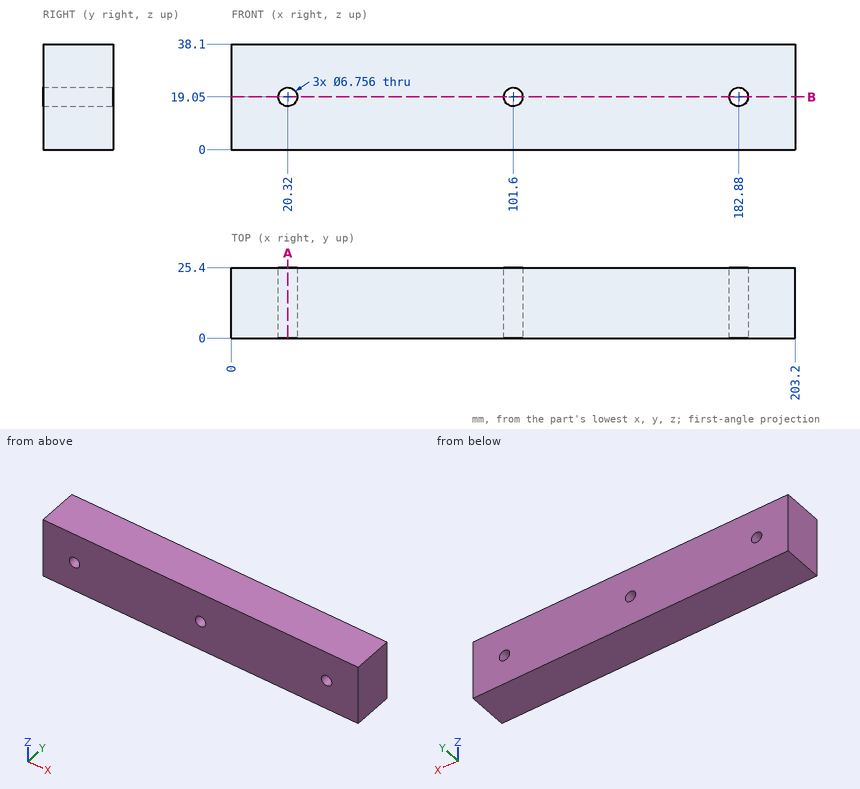
Job drawing, mm, ordinate dimensions from the low corner. One solid piece. Coordinates: 2 decimals unless noted, no trailing zeros. Order: outer loops, then holes, each group sorted by start corner. A loop starts at its lowest first (then second) coordinate and runs counter-clockwise, first axis right, second up. Notation, with made-up numbers: (46, 82) - (58, 82) arc R19 ccw to (58, 99) - close; hole circle Ø1 at (33, 53.25). An arc over 180 degrees is marked (long way). Return JSON: item names as keys, results as strings. Group by question number.
1) Probe line 1 (X direction, y = 13.25, z = 19.05); line 2 (Z direction, x = 20.32, y = 10); line 3 (X direction, y = 16.75, z = 21). List the from-to ranges inside material, lowest first. Write a range as from..to.
2) Saw through at B-B, the plane z = 19.05. Write the cut outline in (x, y), plus the area to 3 significant figures.
3) Saw through at A-A, the plane x = 20.32. Write the cut outline in (y, z).
4) Flat gauge pins, fed straight in: P1, Ø1.5, axis at x = 143.5, y = 3, coming from the -Z side; P2, Ø4, axis at x = 20.32, z = 19.05, coming from the -Y side. Where does each tip first touch, or does it go through?
Values found:
{
 "1": {"line 1": "x = 0..16.94, 23.7..98.22, 104.98..179.5, 186.26..203.2", "line 2": "z = 0..15.67, 22.43..38.1", "line 3": "x = 0..17.56, 23.08..98.84, 104.36..180.12, 185.64..203.2"},
 "2": {"outline": "(0, 0) - (16.94, 0) - (16.94, 25.4) - (0, 25.4) - close; (23.7, 0) - (98.22, 0) - (98.22, 25.4) - (23.7, 25.4) - close; (104.98, 0) - (179.5, 0) - (179.5, 25.4) - (104.98, 25.4) - close; (186.26, 0) - (203.2, 0) - (203.2, 25.4) - (186.26, 25.4) - close", "area": "4,650 mm²"},
 "3": {"outline": "(0, 0) - (25.4, 0) - (25.4, 15.67) - (0, 15.67) - close; (0, 22.43) - (25.4, 22.43) - (25.4, 38.1) - (0, 38.1) - close"},
 "4": {"P1": "stops at z = 0", "P2": "passes through"}
}
